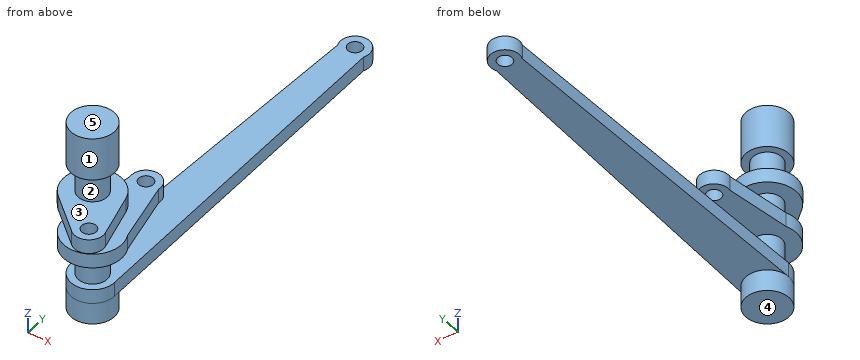
from build123d import *

# Parameters (mm, degrees)
ESBO_O1_R                  = 15
RESSALTO_EXTRUS_O1_DEPTH   = 15
RESSALTO_EXTRUS_O2_DEPTH   = 10
ESBO_O4_R                  = 10
RESSALTO_EXTRUS_O3_DEPTH   = 20
CORTE_EXTRUS_O3_DEPTH      = 262.629509039
CORTE_EXTRUS_O3_DEPTH_BACK = 262.629509039
ESBO_O9_R                  = 5
RESSALTO_EXTRUS_O6_DEPTH   = 10
CORTE_EXTRUS_O4_DEPTH      = 267.505159425
CORTE_EXTRUS_O4_DEPTH_BACK = 10
ESBO_O12_R                 = 5
ESBO_O13_R                 = 10
RESSALTO_EXTRUS_O7_DEPTH   = 20
ESBO_O14_R                 = 5
RESSALTO_EXTRUS_O8_DEPTH   = 10
ESBO_O15_R                 = 10
RESSALTO_EXTRUS_O9_DEPTH   = 20
ESBO_O17_R                 = 15
RESSALTO_EXTRUS_O10_DEPTH  = 30


with BuildPart() as part:
    # Esboço1 → Ressalto-extrusão1 (new body)
    with BuildSketch(Plane.XY):
        Circle(ESBO_O1_R)
    extrude(amount=RESSALTO_EXTRUS_O1_DEPTH)

    # Esboço2 → Ressalto-extrusão2 (add)
    with BuildSketch(Plane.XY.offset(15)):
        with BuildLine():
            Line((-9.078599197, 245.807263828), (-14.995643171, 0.361505045))
            ThreePointArc((-14.995643171, 0.361505045), (-0.00084936, -14.999999976), (14.995684014, 0.359806815))
            Line((14.995684014, 0.359806815), (9.105027046, 245.864968865))
            ThreePointArc((9.105027046, 245.864968865), (-0.031734455, 259.999949646), (-9.078599197, 245.807263828))
        make_face()
    extrude(amount=RESSALTO_EXTRUS_O2_DEPTH)

    # Esboço4 → Ressalto-extrusão3 (add)
    with BuildSketch(Plane.XY.offset(25)):
        Circle(ESBO_O4_R)
    extrude(amount=RESSALTO_EXTRUS_O3_DEPTH)

    # Esboço9 → Corte-extrusão3 (cut, two sides: drawn at the far end of the back side and taken through both)
    with BuildSketch(Plane.XY.offset(25).offset(-CORTE_EXTRUS_O3_DEPTH_BACK)):
        with Locations((0, 250)):
            Circle(ESBO_O9_R)
    extrude(amount=CORTE_EXTRUS_O3_DEPTH + CORTE_EXTRUS_O3_DEPTH_BACK, mode=Mode.SUBTRACT)

    # Esboço11 → Ressalto-extrusão6 (add)
    with BuildSketch(Plane(origin=(0, 0, 45), x_dir=(0.999001995685138, 0.044665564108286114, 0), z_dir=(0, 0, 1))):
        with BuildLine():
            Line((-9.890512739, 52.704277206), (-18.232895862, 8.219580797))
            ThreePointArc((-18.232895862, 8.219580797), (0.107287246, -19.999712234), (18.143662158, 8.414720642))
            Line((18.143662158, 8.414720642), (9.830225014, 52.345149552))
            ThreePointArc((9.830225014, 52.345149552), (0.182076414, 64.178342272), (-9.890512739, 52.704277206))
        make_face()
    extrude(amount=RESSALTO_EXTRUS_O6_DEPTH)

    # Esboço12 → Corte-extrusão4 (cut, two sides: drawn at the far end of the back side and taken through both)
    with BuildSketch(Plane.XY.offset(55).offset(-CORTE_EXTRUS_O4_DEPTH_BACK)):
        with Locations(Location((-2.419980263, 54.125928126, 0), (0, 0, 180))):
            Circle(ESBO_O12_R)
    extrude(amount=CORTE_EXTRUS_O4_DEPTH + CORTE_EXTRUS_O4_DEPTH_BACK, mode=Mode.SUBTRACT)

    # Esboço13 → Ressalto-extrusão7 (add)
    with BuildSketch(Plane.XY.offset(55)):
        Circle(ESBO_O13_R)
    extrude(amount=RESSALTO_EXTRUS_O7_DEPTH)

    # Esboço14 → Ressalto-extrusão8 (add)
    with BuildSketch(Plane(origin=(0, 0, 75), x_dir=(-0.8401882150112437, -0.5422949044166098, 0), z_dir=(0, 0, 1))):
        with BuildLine():
            Line((-9.556625494, 36.904640754), (-19.113250988, 5.889281508))
            ThreePointArc((-19.113250988, 5.889281508), (0, -20), (19.113250988, 5.889281508))
            Line((19.113250988, 5.889281508), (9.556625494, 36.904640754))
            ThreePointArc((9.556625494, 36.904640754), (0, 43.96), (-9.556625494, 36.904640754))
        make_face()
        with Locations(Location((0, 33.96, 0), (0, 0, 147.16))):
            Circle(ESBO_O14_R, mode=Mode.SUBTRACT)
    extrude(amount=RESSALTO_EXTRUS_O8_DEPTH)

    # Esboço15 → Ressalto-extrusão9 (add)
    with BuildSketch(Plane.XY.offset(85)):
        Circle(ESBO_O15_R)
    extrude(amount=RESSALTO_EXTRUS_O9_DEPTH)

    # Esboço17 → Ressalto-extrusão10 (add)
    with BuildSketch(Plane.XY.offset(105)):
        with Locations(Location((0, 0, 0), (0, 0, 178.619018737))):
            Circle(ESBO_O17_R)
    extrude(amount=RESSALTO_EXTRUS_O10_DEPTH)


solid = part.part
CAD build for the part. Positions are in the model's coordinates, mm. Face numbers are marked on the shaded views. A direction names the side the tool comes from. Round coordinates to 2 decimals unless told otherwise and drop trailing zeros. Write each loop counter-clockwise with the first axis right and the second up, starting at its lowest first coordinate (ties: lowest second). Pieces come first, ordered by that corner, then holes.
(1) Slice it at B-B, the plane z = 79. Write the cut outline in (x, y) (3 decimals), and give its area (3 significant figures).
(2) Mould opens along Z. For the marked faces 3, 4 and 5 say: pulls with the +Z half, pulls with the -Z half, needs draft (parallel to the pull), parting line crosses it, or undercut.
(3) Slice it at D-D, the plane y = 27.5. Write the cut outline in (x, z), and give its area (3 significant figures).
(4) Drop flat-ended pins along their axis: P1, Ø3, axis at x = 10.5, y = 157.5, coming from the -Z side; P2, Ø2, axis at x = -7.5, y = 89, coming from the +Z side; P3, Ø10, axis at x = -10.5, y = 40.5, coming from the +Z side. Give the stop position or say it passes through.
(5) Slice it at A-A, the plane y = 250. Write the cut outline in (x, z).
(6) Slice it at C-C, the plane z = 36.5. Write the cut outline in (x, y).
(7) 3-axis set-ups, long thin cutter, end or side, ignore diameter. For the marked faces 1 and 2: which of +Z, -Z, +X, -X, +Y, -Y reach the whole face in a straight line?
(8) Probe line 1 along Z through (x, y) = (3, 42.5); line 2 along Y through (x, z) = (0, 18); line 3 along X through (y, z) = (250, 17.5). List the from-to ranges inside material, lowest first.
From the geometry:
1. outline: (-12.865, -15.313) - (11.984, -36.189) arc R10 ccw to (28.043, -25.824) - (19.252, 5.417) arc R20 ccw (long way) to start; hole circle Ø10 at (18.416, -28.533)
1. area: 1,770 mm2
2. face 3: undercut
2. face 4: pulls with the -Z half
2. face 5: pulls with the +Z half
3. outline: (-15.73, 45) - (13.44, 45) - (13.44, 55) - (-15.73, 55) - close; (-14.34, 15) - (14.34, 15) - (14.34, 25) - (-14.34, 25) - close
3. area: 579 mm2
4. P1: stops at z = 15
4. P2: stops at z = 25
4. P3: stops at z = 55
5. outline: (-10, 15) - (-5, 15) - (-5, 25) - (-10, 25) - close; (5, 15) - (10, 15) - (10, 25) - (5, 25) - close
6. outline: circle Ø20 at (0, 0)
7. face 1: +Z
7. face 2: none
8. line 1: z = 15 to 25, 45 to 55
8. line 2: y = -15 to 245, 255 to 260
8. line 3: x = -10 to -5, 5 to 10
